Verification items for the finished model (mm, model axes). A direction names the side the tool comes from. Coordinates: 2 decimals unless noted, no trailing zeros. Loops run counter-clockwise (first coordinate to the right, second up) from the corner with the lowest first, then second, coordinate; pieces in that order, holes last.
Q1. Sectioned sample at B-B (y = 6). Count the separate pieces of the cut face and the enclosed holes in it, then the cut area to 3 significant figures.
Q2. Mould release check, pull along Z, two halves, no side actions. Record for faces 4 (the face through (-11.7, 1.521, 39.046)), 5 (the face through (-15, 0, 39)), 6 (the face through (-7.234, 6.655, 2.468)), 7 (the face through (-14.28, 8.63, 41.3)): +Z half, -Z half, draft (parallel to the pull), parting line (faces both ways), or undercut.
Q3. Access from +Z, -Z, +X, -X, +Y, -Y to the whole of each face (thin tool, end or side, straight path). Record for faces 1 (the face through (-15.055, 4.056, 42.432)), 2 (the face through (-15, 7, 80)), 3 (the face through (-11.8, 4.76, 41.98)).
Q4. Sectioned sample at A-A (z = 14). Enter the section's corners in (x, y).
Q5. Go/stop test with flat-tipped pins: P1, Ø8, axis at x = -8.5, y = 8.5, coming from the -Z side; P2, Ø1.5, axis at x = -19, z = 40, coming from the -Y side; P3, Ø4, axis at x = -8.5, y = 9, coming from the +Z side; P4, Ø1.6, axis at x = -11.4, z = 40, coming from the -Y side. Record where each tip stops, or that it passes through.
Q6. Material ranges on probe 1 along X at (y, z) = (1.6, 40); probe 2 along Y at (x, z) = (-7.75, 32.5); probe 3 along Z at (x, y) = (-14.2, 5.75), recorded low to high.
Autodesk Fusion 360 part; units mm, degrees
sketch "Sketch1" plane through (0, 0, 0) normal (0, 1, 0) x (1, 0, 0)
  line L0 (0, 0) -> (-24, 0)
  line L1 (-24, 0) -> (-24, -80)
  line L2 (-24, -80) -> (0, -80)
  line L3 (0, -80) -> (0, 0)
  line L4 (-2.4, -80) -> (-2.4, 0) construction
  line L5 (-12.6, 0) -> (-12.6, -80) construction
  line L6 (-22.05, 0) -> (-22.05, -80) construction
  line L7 (-15.95, 0) -> (-15.95, -80) construction
  line L8 (-12.6, -40) -> (-2.4, -40) construction
  line L9 (-7.5, -40) -> (-7.5, 0) construction
  line L10 (-22.05, -40) -> (-15.95, -40) construction
  line L11 (-22.05, -40) -> (-24, -40) construction
  line L12 (-2.4, -40) -> (0, -40) construction
  line L13 (-12.6, -5) -> (-2.4, -5) construction
  line L14 (-14.2, -41.5) -> (-11.4, -41.5) construction
  line L15 (-11.4, -41.5) -> (-11.4, -40) construction
  line L16 (-11.4, -40) -> (-14.2, -40) construction
  line L17 (-14.2, -40) -> (-14.2, -41.5) construction
  point P0 (-19, -40)
  point P1 (-14.2, -41.5)
  point P2 (-11.4, -40)
  dimension "d1" = 24
  dimension "d2" = 80
  dimension "d3" = 10.2
  dimension "d5" = 6.1
  dimension "d7" = 5
  dimension "d8" = 7.5
  dimension "d9" = 75
  dimension "d12" = 1.5
  dimension "d13" = 2.8
  dimension "d14" = 1.2
extrude "Extrude1" add sketch "Sketch1" along normal blind 15
sketch "Sketch2" plane through (0, 0, 80) normal (0, 0, 1) x (-1, 0, 0)
  line L0 (24, 0) -> (0, 0)
  line L1 (0, 0) -> (0, -15)
  line L2 (0, -15) -> (24, -15)
  line L3 (24, -15) -> (24, 0)
  line L4 (15.95, 0) -> (15.95, -15) construction
  line L5 (22.05, 0) -> (22.05, -15) construction
  line L6 (12.6, 0) -> (12.6, -15) construction
  line L7 (2.4, 0) -> (2.4, -15) construction
  line L8 (12.6, -7.5) -> (2.4, -7.5) construction
  line L9 (15.95, -6) -> (22.05, -6) construction
  circle A0 centre (7.5, -7.5) radius 5.1
  circle A1 centre (19, -6) radius 3.05
  point P0 (22.05, 0)
  point P1 (15.95, 0)
  point P2 (12.6, 0)
  point P3 (2.4, 0)
  point P4 (19, 0)
  dimension "d15" = 6
extrude "Extrude2" cut sketch "Sketch2" against normal through all contours A1
hole "Hole1" at (-7.5, 7.5, 80) direction (0, 0, -1) diameter 10.2 depth 75 tip angle 118
hole "Hole2" at (-14.2, 0, 41.5) direction (0, 1, 0) diameter 2.529 depth 8 tip angle 118
hole "Hole3" at (-19, 0, 40) direction (0, 1, 0) diameter 2.529 depth 6 tip angle 118
hole "Hole4" at (-11.4, 0, 40) direction (0, 1, 0) diameter 2 depth 3 tip angle 118
Geometry check:
1. separate pieces: 2
1. enclosed holes: 1
1. area: 683 mm2
2. face 4: undercut
2. face 5: draft
2. face 6: +Z half
2. face 7: undercut
3. face 1: -Y
3. face 2: +Z, +X, -X, +Y, -Y
3. face 3: +Z
4. outline: (-24, 0) - (0, 0) - (0, 15) - (-24, 15) - close; hole circle Ø6.1 at (-19, 6); hole circle Ø10.2 at (-7.5, 7.5)
5. P1: stops at z = 0
5. P2: stops at y = 8.96
5. P3: stops at z = 4.22
5. P4: stops at y = 3.12
6. probe 1: x = -24 to -20.26, -17.74 to -12.4, -10.4 to 0
6. probe 2: y = 0 to 2.41, 12.59 to 15
6. probe 3: z = 0 to 40.24, 42.76 to 80
